Part model, mm, in its own coordinate system. A direction names the side the tool comes from. Give positions to 0.01 mm unless a question says otherwise; leave off trailing zeros. Write each loop counter-clockwise with the first axis right and the second up, starting at its lowest first coordinate (ties: lowest second). Pieces come first, ordered by that corner, then holes. Notation, with made-up numbers: M -11.5,70.5 L 38.5,70.5 A13 ccw 38.5,86.5 Z; hole C -37,7.25 d8. An arc over 180 degrees is marked long. Use a Markdown table: item, result. Add a question column.
from build123d import *

# Parameters (mm, degrees)
BOSS_EXTRUDE2_DEPTH = 15.875
CHAMFER1_SIZE       = 3.175


with BuildPart() as part:
    # Sketch3 → Boss-Extrude2 (new, symmetric)
    with BuildSketch(Plane(origin=(0, 0, 0), x_dir=(0, 0, -1), z_dir=(1, 0, 0))):
        with BuildLine():
            ThreePointArc((3.1877, 9.525), (-2.433940332, 7.196440332), (-4.7625, 1.5748))
            Line((-4.7625, 1.5748), (-4.7625, -9.525))
            Line((-4.7625, -9.525), (4.7625, -9.525))
            Line((4.7625, -9.525), (4.7625, 9.525))
            Line((4.7625, 9.525), (3.1877, 9.525))
        make_face()
    extrude(amount=BOSS_EXTRUDE2_DEPTH, both=True)

    # Chamfer1
    chamfer1_edges = [part.edges().sort_by_distance(p)[0] for p in [
        (15.875, -9.525, 0),
        (-15.875, -9.525, 0),
    ]]
    chamfer(chamfer1_edges, length=CHAMFER1_SIZE)

    # Sketch4 → Cut-Revolve2 (revolve, cut)
    with BuildSketch(Plane(origin=(0, 0, 0), x_dir=(0, 0, -1), z_dir=(1, 0, 0)), mode=Mode.PRIVATE) as cut_revolve2_sk:
        Polygon((-4.7625, 4.09575), (0.8001, 4.09575), (0.8001, 5.6769), (4.7625, 5.6769), (4.7625, 0), (-4.7625, 0), align=None)
    revolve(cut_revolve2_sk.sketch.rotate(Axis((0, 0, 4.7625), (0, 0, -1)), 180), axis=Axis((0, 0, 4.7625), (0, 0, -1)), mode=Mode.SUBTRACT)


solid = part.part
1. Cut at B-B (z = -1.75). Write the cut outline in (x, y) (3 decimals), then the cut area to 3 significant figures.
2. Tool access for faces 1 (the cylindrical face through (-1.23, -3.907, 1.942)), 2 (the cylindrical face through (-5.63, 0.74, -2.81)): list every direction of +Z, -Z, +X, -X, +Y, -Y with a clear straight run to the whole face (end or side of a thin tool).
3. Cut at D-D (x = 7.5). Write the cut outline in (y, z) (1 decimal), then the cut area to 3 significant figures.
4. Cut at A-A (y = 0). Write the cut outline in (x, z) (1 decimal), then the cut area to 3 significant figures.
5. Cut at C-C (x = 0). Write the cut outline in (y, z) (1 decimal).
6. Drill centre lines: probe 1 along X at (y, z) = (0, -3) (3 decimals); probe 2 along X at (y, z) = (0, 2.7) (3 decimals); probe 3 along Y at (x, z) = (2.5, 0) (3 decimals). Where is each one in solid material? Low to high. Write a range as [from, to].
7. Flat gauge pins, fed straight in: pin 1 (9 mm diameter, centred on x = 0, y = 0, fed in from -Z); pin 2 (1.5 mm diameter, centred on x = 2.5, y = 5.5, fed in from +Z). Where does each tip first touch, or does it go through?
A:
| question | item | result |
|---|---|---|
| 1 | outline | M -15.875,-6.35 L -12.7,-9.525 L 12.7,-9.525 L 15.875,-6.35 L 15.875,9.394 L -15.875,9.394 Z; hole C 0,0 d11.354 |
| 1 | area | 489 mm² |
| 2 | face 1 | +Z, -Z |
| 2 | face 2 | -Z |
| 3 | outline | M -9.5,-4.8 L 9.5,-4.8 L 9.5,-3.2 A8 ccw 1.6,4.8 L -9.5,4.8 Z |
| 3 | area | 168 mm² |
| 4 | outline | M -15.9,-4.8 L -5.7,-4.8 L -5.7,-0.8 L -4.1,-0.8 L -4.1,4.8 L -15.9,4.8 Z; M 4.1,-0.8 L 5.7,-0.8 L 5.7,-4.8 L 15.9,-4.8 L 15.9,4.8 L 4.1,4.8 Z |
| 4 | area | 212 mm² |
| 5 | outline | M -9.5,-4.8 L -5.7,-4.8 L -5.7,-0.8 L -4.1,-0.8 L -4.1,4.8 L -9.5,4.8 Z; M 4.1,-0.8 L 5.7,-0.8 L 5.7,-4.8 L 9.5,-4.8 L 9.5,-3.2 A8 ccw 4.1,4.4 Z |
| 6 | probe 1 | x = [-15.875, -5.677], [5.677, 15.875] |
| 6 | probe 2 | x = [-15.875, -4.096], [4.096, 15.875] |
| 6 | probe 3 | y = [-9.525, -3.244], [3.244, 8.858] |
| 7 | pin 1 | stops at z = -0.8 |
| 7 | pin 2 | stops at z = 4.1 |
